Part print with two shaded views. Sizes in mm from the minimum x, y, z corner. A direction names the side the tool comes from. Round coordinates to 2 decimals unless told otherwise and drop trailing zeros. Write each loop counter-clockwise with the first axis right and the second up, starting at its lowest first coordinate (ties: lowest second). Pieces come first, ordered by that corner, then holes. Notation, with made-up numbers: (54, -17) - (62, -17) arc R17 ccw to (62, 3) - close; hole circle Ø2 at (78.5, 31). An arc over 180 degrees is marked (long way). Use one line per item in the form item = value. Start each with the question number.
Item 1: Tool access for the marked faces 4, 5 and 6: list every direction of +Z, -Z, +X, -X, +Y, -Y with a clear straight run to the whole face (end or side of a thin tool).
Item 2: Pin check, flat tips, straight feed: pin 1 (1 mm diameter, centred on y = 21, z = 1, fed in from +X); pin 2 (0.7 mm diameter, centred on x = 22, y = 23, fed in from +Z); pin 3 (2 mm diameter, centred on x = 27.5, z = 1.5, fed in from +Y); pin 4 (18.5 mm diameter, centred on x = 18, y = 17, fed in from +Z). Stop position of each tip, or through.
Item 3: Band-saw the part on B-B, the plane z = 5.75. List the corners of the cut face in (x, y), and give its area (3 significant figures).
Item 4: Drill centre lines: L1, parallel to Y at x = 22.5, z = 3.8 (3 decimals); L2, parallel to Y at x = 22.5, z = 5.2; L3, parallel to X at y = 20, z = 5. Where is each one in solid material? Low to high.
Item 5: Pull direction Z, two halves, no side cores. Call the marked faces 1, 2 and 3: +Z half, -Z half, draft (parallel to the pull), parting line (faces both ways), or undercut.
Item 6: Band-saw the part on A-A, the plane y = 22.5. List the corners of the cut face in (x, z).
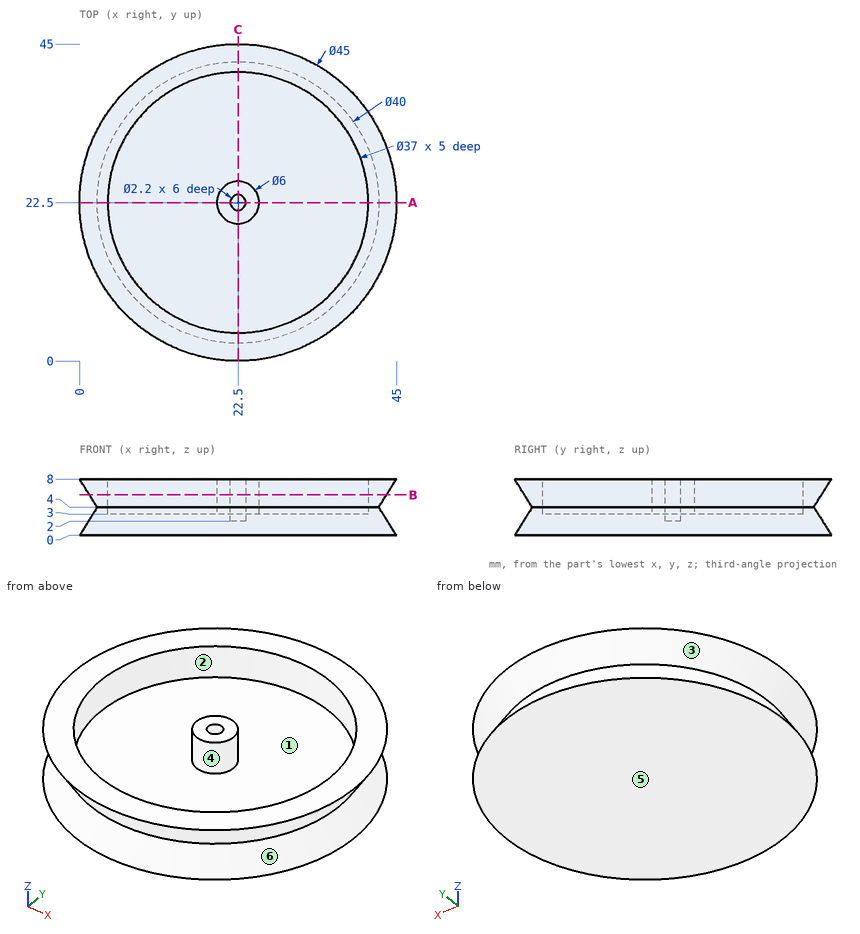
Determined:
q1.face_4 = +Z
q1.face_5 = -Z, +X, -X, +Y, -Y
q1.face_6 = none
q2.pin_1 = 44.64
q2.pin_2 = 2
q2.pin_3 = 44.15
q2.pin_4 = 8
q3.outline = circle Ø42.19 at (22.5, 22.5); circle Ø6 at (22.5, 22.5); hole circle Ø37 at (22.5, 22.5); hole circle Ø2.2 at (22.5, 22.5)
q3.area = 347 mm²
q4.L1 = 2.375 to 4, 19.5 to 21.4, 23.6 to 25.5, 41 to 42.625
q4.L2 = 1.75 to 4, 19.5 to 21.4, 23.6 to 25.5, 41 to 43.25
q4.L3 = 2.03 to 4.17, 20.84 to 24.16, 40.83 to 42.97
q5.face_1 = +Z half
q5.face_2 = draft
q5.face_3 = undercut
q6.outline = (0, 0) - (45, 0) - (42.5, 4) - (45, 8) - (41, 8) - (41, 3) - (25.5, 3) - (25.5, 8) - (23.6, 8) - (23.6, 2) - (21.4, 2) - (21.4, 8) - (19.5, 8) - (19.5, 3) - (4, 3) - (4, 8) - (0, 8) - (2.5, 4) - close
